Geometry check sheet. Reference: the model listing, model coordinates, mm. Round coordinates to 2 decimals unless told otherwise and drop trailing zeros. Order: outer loops, then holes, each group sorted by start corner. A loop starts at its lowest first (then second) coordinate and runs counter-clockwise, first axis right, second up.
(1) Sectioned sample at B-B (z = 39). Record the boundary of the cut face in (x, y).
(2) Sectioned sample at C-C (y = 582.5). Record the boundary of the cut face in (x, z), plus the area to 3 significant figures.
(3) Go/stop test with flat-tipped pins: pin 1 (5.5 mm diameter, centred on x = 13.5, y = 499.5, fed in from -Z); pin 2 (5.5 mm diameter, centred on x = 6.5, z = 179, fed in from +Y); pin 3 (1.5 mm diameter, centred on x = 9.5, z = 271.5, fed in from -Y); pin 4 (9.5 mm diameter, centred on x = 8, z = 251.5, fed in from +Y). Record where each tip stops, or that it passes through.
(4) Sectioned sample at A-A (x = 3.75). Record the boundary of the cut face in (y, z), plus the area to 3 significant figures.
(5) Material ranges on line 1 along Z through (x, y) = (8.75, 250.5); line 2 along Y through (x, z) = (3.75, 226); line 3 along Z through (x, y) = (13.75, 370.5), recorded low to high.
from build123d import *

# Parameters (mm, degrees)
F0_W     = 254
F0_H     = 387.35
F1_DEPTH = 19.05
F2_W     = 12.7
F2_H     = 146.05
F3_DEPTH = 19.051
F4_W     = 723.9
F4_H     = 127
F5_DEPTH = 19.05


with BuildPart() as f1:
    # F0 (on Right) → F1 (new body)
    with BuildSketch(Plane.YZ):
        with Locations((127, 193.675)):
            Rectangle(F0_W, F0_H)
    extrude(amount=F1_DEPTH)

    # F2 (on face) → F3 (cut, through all)
    with BuildSketch(Plane.YZ.offset(19.05)):
        with Locations((247.65, 314.325)):
            Rectangle(F2_W, F2_H)
    extrude(amount=-F3_DEPTH, mode=Mode.SUBTRACT)

    # F4 (on face) → F5 (join)
    with BuildSketch(Plane.YZ.offset(19.05)):
        with Locations((603.25, 323.85)):
            Rectangle(F4_W, F4_H)
    extrude(amount=-F5_DEPTH)


solid = f1.part
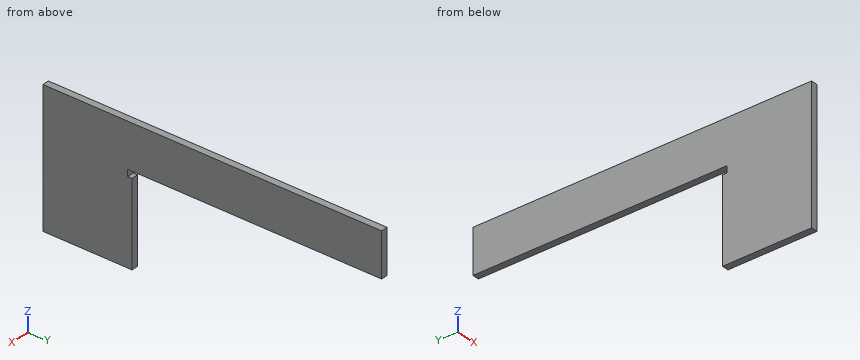
Answer below:
1. outline: (0, 0) - (19.05, 0) - (19.05, 254) - (0, 254) - close
2. outline: (0, 260.35) - (19.05, 260.35) - (19.05, 387.35) - (0, 387.35) - close
2. area: 2,420 mm2
3. pin 1: stops at z = 260.35
3. pin 2: stops at y = 254
3. pin 3: stops at y = 0
3. pin 4: stops at y = 241.3
4. outline: (0, 0) - (254, 0) - (254, 241.3) - (241.3, 241.3) - (241.3, 260.35) - (965.2, 260.35) - (965.2, 387.35) - (0, 387.35) - close
4. area: 188,000 mm2
5. line 1: z = 0 to 241.3, 260.35 to 387.35
5. line 2: y = 0 to 254
5. line 3: z = 260.35 to 387.35
